CAD build for the part. Positions are in the model's coordinates, mm. A direction names the side the tool comes from. Round coordinates to 2 decimals unless told otherwise and drop trailing zeros. Write each loop counter-clockwise with the first axis right and the second up, starting at its lowest first coordinate (ties: lowest second). Pieces come first, ordered by that corner, then holes. Notation, with made-up numbers: (63, 71) - (94, 71) arc R17 cw to (94, 78) - close; hole circle Ø7 at (64.5, 12). An arc over 180 degrees is marked (long way). Answer in a Markdown table with one row per item.
```python
from build123d import *
from OCP.BRepFilletAPI import BRepFilletAPI_MakeChamfer

# Parameters (mm, degrees)
BOSS_EXTRUDE1_START      = -0.01
BOSS_EXTRUDE1_DEPTH      = 3.5
CUT_EXTRUDE1_DEPTH       = 2.925
SKETCH5_R                = 1.5
SKETCH5_R_2              = 1.375
SKETCH5_W                = 7
SKETCH5_H                = 2.5
SKETCH5_H_2              = 3
BOSS_EXTRUDE2_DEPTH      = 2.45
CHAMFER1_SIZE            = 1
CHAMFER1_SIZE_2          = 2.475086853
SKETCH15_R               = 0.75
BOSS_EXTRUDE5_DEPTH      = 0.465
SKETCH7_W                = 7.65
SKETCH7_H                = 2.45
CUT_EXTRUDE2_DEPTH       = 3
BOSS_EXTRUDE3_START      = 0.01
BOSS_EXTRUDE3_DEPTH      = 3.465
CUT_EXTRUDE3_DEPTH       = 2.475
SKETCH10_R               = 1.5
SKETCH10_R_2             = 1.375
BOSS_EXTRUDE4_DEPTH      = 2
CHAMFER2_SIZE            = 0.5
CHAMFER2_SIZE_2          = 2
BOSS_EXTRUDE6_START      = 2.95
SKETCH10_3_R             = 0.75
BOSS_EXTRUDE6_DEPTH      = 2.95
SKETCH21_W               = 2
SKETCH21_H               = 15.4
BOSS_EXTRUDE7_DEPTH      = 2
CUT_EXTRUDE6_START       = -3.465
SKETCH16_R               = 1
CUT_EXTRUDE6_DEPTH       = 38.860351794
SKETCH19_R               = 0.8
CUT_EXTRUDE9_DEPTH       = 35.395351794
SKETCH17_R               = 1.85
CUT_EXTRUDE7_DEPTH       = 2
SKETCH12_W               = 5
SKETCH12_H               = 4.8
CUT_EXTRUDE4_DEPTH       = 1
SKETCH13_R               = 1.475
CUT_EXTRUDE5_DEPTH       = 11.91309
CUT_EXTRUDE10_START      = -23
CUT_EXTRUDE10_DEPTH      = 9
CUT_EXTRUDE10_START_2    = -13.91308954
CUT_EXTRUDE10_2_DEPTH    = 2
CUT_EXTRUDE11_DEPTH      = 35.395351794
CUT_EXTRUDE11_DEPTH_BACK = 35.395351794
SKETCH22_W               = 1.5
SKETCH22_H               = 12
SKETCH22_W_2             = 43.847191308
SKETCH22_H_2             = 1.5
FILLET1_R                = 1.5
FILLET2_R                = 1.5
FILLET3_R                = 1
FILLET4_R                = 1


with BuildPart() as part:
    # Sketch2 → Boss-Extrude1 (new body)
    with BuildSketch(Plane(origin=(0, 0, 0), x_dir=(1, 0, 0), z_dir=(0, 1, 0)).offset(BOSS_EXTRUDE1_START)):
        Polygon((-23, 10.5), (21.303656906, 10.5), (26.250323572, 5.2), (32, 5.2), (32, -5.2), (26.250323572, -5.2), (21.303656906, -10.5), (-23, -10.5), align=None)
    extrude(amount=-BOSS_EXTRUDE1_DEPTH)

    # Sketch3 → Cut-Extrude1 (cut)
    with BuildSketch(Plane(origin=(0, 0, 0), x_dir=(1, 0, 0), z_dir=(0, 1, 0))):
        Polygon((-20.2, 7.7), (-20.2, -7.7), (20.08691046, -7.7), (27.273577127, 0), (20.08691046, 7.7), align=None)
    extrude(amount=-CUT_EXTRUDE1_DEPTH, mode=Mode.SUBTRACT)

    # Sketch5 → Boss-Extrude2 (add)
    with BuildSketch(Plane(origin=(0, -2.925, 0), x_dir=(1, 0, 0), z_dir=(0, 1, 0))):
        with Locations(Location((-11, -5, 0), (0, 0, 270))):
            Circle(SKETCH5_R)
        with Locations(Location((15.125, 5.125, 0), (0, 0, 270))):
            Circle(SKETCH5_R_2)
        with Locations((-16.7, -6.45)):
            Rectangle(SKETCH5_W, SKETCH5_H)
        with Locations((-16.7, 6.45)):
            Rectangle(SKETCH5_W, SKETCH5_H)
        with Locations((13.5, 0)):
            Rectangle(SKETCH5_W, SKETCH5_H_2)
    extrude(amount=BOSS_EXTRUDE2_DEPTH)

    # Chamfer1
    # the kernel refuses this chamfer: 2.475086853, 1 mm, written as the material it adds along each edge
    with BuildSketch(Plane(origin=(-11, -2.925, 5), x_dir=(0, 0, 1), z_dir=(-1, 0, 0))) as chamfer1_piece_1_section:
        Polygon((1.5 + CHAMFER1_SIZE, 0), (1.5, CHAMFER1_SIZE_2), (1.5, 0), align=None)
    chamfer1_piece_1 = revolve(axis=Axis((-11, -2.925, 5), (0, 1, 0)), mode=Mode.PRIVATE)
    chamfer1_piece_1 = split(chamfer1_piece_1, bisect_by=Plane(origin=(-11, -0.475, 5), z_dir=(0, -1, 0)), keep=Keep.TOP, mode=Mode.PRIVATE)
    add(chamfer1_piece_1)
    with BuildSketch(Plane(origin=(15.125, -2.925, -5.125), x_dir=(0, 0, 1), z_dir=(-1, 0, 0))) as chamfer1_piece_2_section:
        Polygon((1.375 + CHAMFER1_SIZE, 0), (1.375, CHAMFER1_SIZE_2), (1.375, 0), align=None)
    chamfer1_piece_2 = revolve(axis=Axis((15.125, -2.925, -5.125), (0, 1, 0)), mode=Mode.PRIVATE)
    chamfer1_piece_2 = split(chamfer1_piece_2, bisect_by=Plane(origin=(15.125, -0.475, -5.125), z_dir=(0, -1, 0)), keep=Keep.TOP, mode=Mode.PRIVATE)
    add(chamfer1_piece_2)

    # Sketch15 → Boss-Extrude5 (add)
    with BuildSketch(Plane(origin=(0, -0.475, 0), x_dir=(1, 0, 0), z_dir=(0, 1, 0))):
        with Locations(Location((-11, -5, 0), (0, 0, 90))):
            Circle(SKETCH15_R)
        with Locations(Location((15.125, 5.125, 0), (0, 0, 90))):
            Circle(SKETCH15_R)
    extrude(amount=BOSS_EXTRUDE5_DEPTH)

    # Sketch7 → Cut-Extrude2 (cut)
    with BuildSketch(Plane.ZY.offset(23)):
        with Locations((0, -1.7)):
            Rectangle(SKETCH7_W, SKETCH7_H)
    extrude(amount=-CUT_EXTRUDE2_DEPTH, mode=Mode.SUBTRACT)

    # Sketch19 → Cut-Extrude9 (cut, through all)
    with BuildSketch(Plane.XZ.offset(3.51)):
        with Locations(Location((-21, -8.5, 0), (0, 0, 270))):
            Circle(SKETCH19_R)
        with Locations(Location((28, -3.2, 0), (0, 0, 270))):
            Circle(SKETCH19_R)
    cut_extrude9 = extrude(amount=-CUT_EXTRUDE9_DEPTH, mode=Mode.SUBTRACT)


with BuildPart() as body_2:
    # Sketch2<2> → Boss-Extrude3 (new body)
    with BuildSketch(Plane(origin=(0, 0, 0), x_dir=(1, 0, 0), z_dir=(0, 1, 0)).offset(BOSS_EXTRUDE3_START)):
        Polygon((-23, 10.5), (21.303656906, 10.5), (26.250323572, 5.2), (32, 5.2), (32, -5.2), (26.250323572, -5.2), (21.303656906, -10.5), (-23, -10.5), align=None)
    extrude(amount=BOSS_EXTRUDE3_DEPTH)

    # Sketch3<2> → Cut-Extrude3 (cut)
    with BuildSketch(Plane(origin=(0, 0, 0), x_dir=(1, 0, 0), z_dir=(0, 1, 0))):
        Polygon((-20.2, 7.7), (-20.2, -7.7), (20.08691046, -7.7), (27.273577127, 0), (20.08691046, 7.7), align=None)
    extrude(amount=CUT_EXTRUDE3_DEPTH, mode=Mode.SUBTRACT)

    # Sketch10 → Boss-Extrude4 (add)
    with BuildSketch(Plane.XZ.offset(-2.475)):
        with Locations(Location((-11, 5, 0), (0, 0, 270))):
            Circle(SKETCH10_R)
        with Locations(Location((15.125, -5.125, 0), (0, 0, 270))):
            Circle(SKETCH10_R_2)
    extrude(amount=BOSS_EXTRUDE4_DEPTH)

    # Chamfer2
    chamfer2_edges_1 = [body_2.edges().sort_by_distance(p)[0] for p in [
        (-11, 2.475, 6.5),
    ]]
    chamfer2_side_1 = [body_2.faces().sort_by_distance(p)[0] for p in [
        (-11, 2.475, 6.51),
    ]]
    chamfer2_edges_2 = [body_2.edges().sort_by_distance(p)[0] for p in [
        (15.125, 2.475, -3.75),
    ]]
    chamfer2_side_2 = [body_2.faces().sort_by_distance(p)[0] for p in [
        (15.125, 2.475, -3.74),
    ]]
    chamfer2 = BRepFilletAPI_MakeChamfer(body_2.part.solid().wrapped)
    for e in chamfer2_edges_1:
        chamfer2.Add(CHAMFER2_SIZE - 0.0001, CHAMFER2_SIZE_2 - 0.0001, e.wrapped, chamfer2_side_1[0].wrapped)
    for e in chamfer2_edges_2:
        chamfer2.Add(CHAMFER2_SIZE - 0.0001, CHAMFER2_SIZE_2 - 0.0001, e.wrapped, chamfer2_side_2[0].wrapped)
    add(Compound.cast(chamfer2.Shape()), mode=Mode.REPLACE)  # a hair under: the kernel refuses the full size

    # Sketch10<3> → Boss-Extrude6 (add)
    with BuildSketch(Plane.XZ.offset(-2.475).offset(BOSS_EXTRUDE6_START)):
        with Locations(Location((-11, 5, 0), (0, 0, 270))):
            Circle(SKETCH10_3_R)
        with Locations(Location((15.125, -5.125, 0), (0, 0, 270))):
            Circle(SKETCH10_3_R)
    extrude(amount=-BOSS_EXTRUDE6_DEPTH)

    # Sketch21 → Boss-Extrude7 (add)
    with BuildSketch(Plane.XZ.offset(-2.475)):
        Polygon((-20.2, 7.7), (-18.2, 7.7), (-18.2, 2), (-14.2, 2), (-14.2, -2), (-18.2, -2), (-18.2, -7.7), (-20.2, -7.7), align=None)
        with Locations((19.08691046, 0)):
            Rectangle(SKETCH21_W, SKETCH21_H)
    extrude(amount=BOSS_EXTRUDE7_DEPTH)

    # Sketch16 → Cut-Extrude6 (cut)
    with BuildSketch(Plane(origin=(0, 3.475, 0), x_dir=(1, 0, 0), z_dir=(0, 1, 0)).offset(CUT_EXTRUDE6_START)):
        with Locations(Location((-21, 8.5, 0), (0, 0, 90))):
            Circle(SKETCH16_R)
        with Locations(Location((28, 3.2, 0), (0, 0, 90))):
            Circle(SKETCH16_R)
    cut_extrude6 = extrude(amount=CUT_EXTRUDE6_DEPTH, mode=Mode.SUBTRACT)

    # Sketch17 → Cut-Extrude7 (cut)
    with BuildSketch(Plane(origin=(0, 3.475, 0), x_dir=(1, 0, 0), z_dir=(0, 1, 0))):
        with Locations(Location((-21, 8.5, 0), (0, 0, 270))):
            Circle(SKETCH17_R)
        with Locations(Location((28, 3.2, 0), (0, 0, 270))):
            Circle(SKETCH17_R)
    cut_extrude7 = extrude(amount=-CUT_EXTRUDE7_DEPTH, mode=Mode.SUBTRACT)


with BuildPart() as mirror2_tool:
    # Mirror2: Cut-Extrude6, Cut-Extrude9, Cut-Extrude7 across plane
    add(cut_extrude6.mirror(Plane.XY))
    add(cut_extrude9.mirror(Plane.XY))
    add(cut_extrude7.mirror(Plane.XY))


with BuildPart() as part_1:
    add(part.part)

    # Mirror2: cut by mirror2_tool
    add(mirror2_tool.part, mode=Mode.SUBTRACT)


with BuildPart() as body_2_1:
    add(body_2.part)

    # Mirror2: cut by mirror2_tool
    add(mirror2_tool.part, mode=Mode.SUBTRACT)

    # Sketch12 → Cut-Extrude4 (cut)
    with BuildSketch(Plane(origin=(0, 3.475, 0), x_dir=(1, 0, 0), z_dir=(0, 1, 0))):
        with Locations((-9.5, -0.5)):
            Rectangle(SKETCH12_W, SKETCH12_H)
    extrude(amount=-CUT_EXTRUDE4_DEPTH, mode=Mode.SUBTRACT)


with BuildPart() as cut_extrude5_tool:
    # Sketch13 → Cut-Extrude5 (new body)
    with BuildSketch(Plane(origin=(32, 0, 0), x_dir=(0, 0, -1), z_dir=(1, 0, 0))):
        Circle(SKETCH13_R)
    extrude(amount=-CUT_EXTRUDE5_DEPTH)


with BuildPart() as part_2:
    add(part_1.part)

    # Cut-Extrude5: cut by cut_extrude5_tool
    add(cut_extrude5_tool.part, mode=Mode.SUBTRACT)

    # Cut-Extrude10: read off the stored shape, not the designer's step
    # Cut-Extrude10 outline → Cut-Extrude10 (cut)
    with BuildSketch(Plane(origin=(32, 0, 0), x_dir=(0, 0, -1), z_dir=(1, 0, 0)).offset(CUT_EXTRUDE10_START)):
        with BuildLine():
            Line((0.504752415, -0.475), (-0.504752415, -0.475))
            ThreePointArc((-0.504752415, -0.475), (0, -0.69), (0.504752415, -0.475))
        make_face()
    extrude(amount=CUT_EXTRUDE10_DEPTH, mode=Mode.SUBTRACT)


with BuildPart() as body_2_2:
    add(body_2_1.part)

    # Cut-Extrude5: cut by cut_extrude5_tool
    add(cut_extrude5_tool.part, mode=Mode.SUBTRACT)

    # Cut-Extrude10 2 outline → Cut-Extrude10 2 (cut)
    with BuildSketch(Plane(origin=(32, 0, 0), x_dir=(0, 0, -1), z_dir=(1, 0, 0)).offset(CUT_EXTRUDE10_START_2)):
        with BuildLine():
            Line((-0.523235129, 0.475), (0.523235129, 0.475))
            ThreePointArc((0.523235129, 0.475), (0, 0.71), (-0.523235129, 0.475))
        make_face()
    extrude(amount=CUT_EXTRUDE10_2_DEPTH, mode=Mode.SUBTRACT)


with BuildPart() as cut_extrude11_tool:
    # Sketch22 → Cut-Extrude11 (new, two sides: drawn at the far end of the back side and taken through both)
    with BuildSketch(Plane(origin=(0, 3.475, 0), x_dir=(1, 0, 0), z_dir=(0, 1, 0)).offset(-CUT_EXTRUDE11_DEPTH_BACK)):
        with Locations((-22.25, 0)):
            Rectangle(SKETCH22_W, SKETCH22_H)
        with Locations((3.423595654, 9.75)):
            Rectangle(SKETCH22_W_2, SKETCH22_H_2)
        with Locations((3.423595654, -9.75)):
            Rectangle(SKETCH22_W_2, SKETCH22_H_2)
    extrude(amount=CUT_EXTRUDE11_DEPTH + CUT_EXTRUDE11_DEPTH_BACK)


with BuildPart() as part_3:
    add(part_2.part)

    # Cut-Extrude11: cut by cut_extrude11_tool
    add(cut_extrude11_tool.part, mode=Mode.SUBTRACT)

    # Fillet2
    fillet2_edges = [part_3.edges().sort_by_distance(p)[0] for p in [
        (-18.5, -1.76, -10.5),
        (-18.5, -1.76, 10.5),
        (-23, -1.76, -6),
        (-23, -1.76, 10.5),
        (32, -1.76, 5.2),
        (-23, -1.76, 6),
        (-23, -1.76, -10.5),
        (32, -1.76, -5.2),
        (22.703656906, -1.76, 9),
        (22.703656906, -1.76, -9),
    ]]
    fillet(fillet2_edges, radius=FILLET2_R - 0.0001)  # a hair under: the kernel refuses the full size

    # Fillet4
    fillet4_edges = [part_3.edges().sort_by_distance(p)[0] for p in [
        (-21.5, -1.76, 6),
        (-21.5, -1.76, -6),
        (-18.5, -1.76, -9),
        (-18.5, -1.76, 9),
    ]]
    fillet(fillet4_edges, radius=FILLET4_R)


with BuildPart() as body_2_3:
    add(body_2_2.part)

    # Cut-Extrude11: cut by cut_extrude11_tool
    add(cut_extrude11_tool.part, mode=Mode.SUBTRACT)

    # Fillet1
    fillet1_edges = [body_2_3.edges().sort_by_distance(p)[0] for p in [
        (-23, 1.7425, -10.5),
        (-23, 1.7425, -6),
        (32, 1.7425, -5.2),
        (32, 1.7425, 5.2),
        (-18.5, 1.7425, 10.5),
        (-23, 1.7425, 6),
        (-23, 1.7425, 10.5),
        (-18.5, 1.7425, -10.5),
        (22.703656906, 1.7425, -9),
        (22.703656906, 1.7425, 9),
    ]]
    fillet(fillet1_edges, radius=FILLET1_R - 0.0001)  # a hair under: the kernel refuses the full size

    # Fillet3
    fillet3_edges = [body_2_3.edges().sort_by_distance(p)[0] for p in [
        (-21.5, 1.7425, -6),
        (-21.5, 1.7425, 6),
        (-18.5, 1.7425, -9),
        (-18.5, 1.7425, 9),
    ]]
    fillet(fillet3_edges, radius=FILLET3_R)


solid = part_3.part
```
Q1. Saw through at C-C on x = 19. List the corners of the cut face in (y, z) (3 decimals).
Computed:
| item | result |
|---|---|
| outline | (-3.51, -9) - (-0.01, -9) - (-0.01, -7.7) - (-2.925, -7.7) - (-2.925, 7.7) - (-0.01, 7.7) - (-0.01, 9) - (-3.51, 9) - close |
Q2. Flat gauge pins, fed straight in: pin 1 (0.9 mm diameter, centred on x = 2.5, y = -1, fed in from +Z); pin 2 (1.2 mm diameter, centred on y = -1, z = 7, fed in from +X); pin 3 (2 mm diameter, centred on y = -1.5, z = -6.5, fed in from +X); pin 4 (1.3 mm diameter, centred on x = -21, z = -8.5, fed in from +Y). Where does each tip first touch, or does it go through?
Computed:
| item | result |
|---|---|
| pin 1 | stops at z = 9 |
| pin 2 | stops at x = 25.13 |
| pin 3 | stops at x = 25.97 |
| pin 4 | passes through |
Q3. Saw through at B-B on x = -11. List the corners of the cut face in (y, z) (3 decimals), then the cut area to 3 significant figures.
Computed:
| item | result |
|---|---|
| outline | (-3.51, -9) - (-0.01, -9) - (-0.01, -7.7) - (-2.925, -7.7) - (-2.925, 2.5) - (-0.475, 3.49) - (-0.475, 4.25) - (-0.01, 4.25) - (-0.01, 5.75) - (-0.475, 5.75) - (-0.475, 6.51) - (-2.925, 7.5) - (-2.925, 7.7) - (-0.01, 7.7) - (-0.01, 9) - (-3.51, 9) - close |
| area | 28.6 mm2 |
Q4. 3-axis set-ups, long thin cutter, end or side, ignore diameter. For faces 1 (the flat face through (23.731, -1.447, -3.796)), 2 (the flat face through (13, -2, -1.5)), 3 (the cylindrical face through (28.991, -1.475, 0.032)): which of +Z, -Z, +X, -X, +Y, -Y reach the whole face in a straight line?
Computed:
| item | result |
|---|---|
| face 1 | +Y |
| face 2 | -X, +Y |
| face 3 | +X, +Y |
Q5. Saw through at A-A on x = 28. List the corners of the cut face in (y, z) (3 decimals), then the cut area to 3 significant figures.
Computed:
| item | result |
|---|---|
| outline | (-3.51, -5.2) - (-0.01, -5.2) - (-0.01, -4) - (-3.51, -4) - close; (-3.51, -2.4) - (-0.01, -2.4) - (-0.01, -1.475) arc R1.475 cw to (-0.01, 1.475) - (-0.01, 2.4) - (-3.51, 2.4) - close; (-3.51, 4) - (-0.01, 4) - (-0.01, 5.2) - (-3.51, 5.2) - close |
| area | 21.8 mm2 |
Q6. Drill centre lines: line 1 (Z direction, x = -11, y = -0.6); line 2 (Z direction, x = -3, y = -2.5); line 3 (Y direction, x = 1.5, z = -1.75) (3 decimals). Where is each one in solid material? Low to high.
Computed:
| item | result |
|---|---|
| line 1 | z = -9 to -7.7, 3.44 to 6.56, 7.7 to 9 |
| line 2 | z = -9 to -7.7, 7.7 to 9 |
| line 3 | y = -3.51 to -2.925 |
Q7. Pull direction X, two halves, no side cores. Call faces 4 (the cylindrical face through (28.675, -1.784, -3.63)), 5 (the flat face through (-21, -0.475, 0)), 6 (the cylindrical face through (-22.75, -1.74, 6.67)): released by +X, released by -X, zero draft, split by the parting line, or undercut.
Computed:
| item | result |
|---|---|
| face 4 | undercut |
| face 5 | zero draft |
| face 6 | released by -X |
